Source: CAD feature listing. Evaluate the final solid. Frame: model axes, mm. Face numbers are marked on the shaded views. A direction names the side the tool comes from. Give positions to 0.01 mm unless a question says otherwise; leave off trailing zeros. Write item = value, one per line.
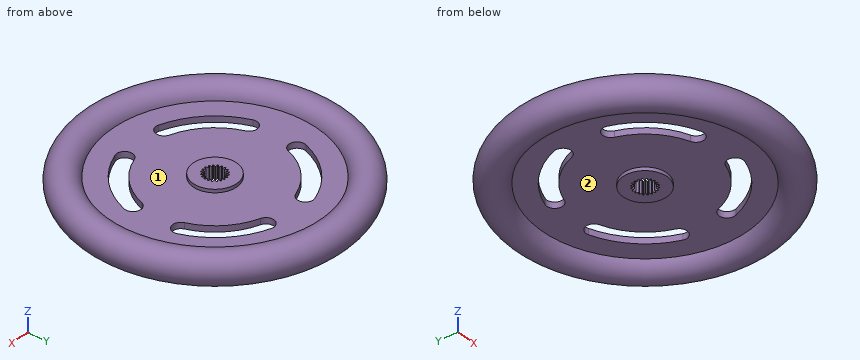
from build123d import *

# Parameters (mm, degrees)
SKETCH2_R                = 3.81
BOSS_EXTRUDE1_DEPTH      = 1.585
BOSS_EXTRUDE1_DEPTH_BACK = 1.585
SKETCH4_R                = 5.485
BOSS_EXTRUDE2_DEPTH      = 0.75
BOSS_EXTRUDE2_DEPTH_BACK = 0.75
SKETCH5_R                = 26.708345462
SKETCH5_R_2              = 4.443835797


with BuildPart() as part:
    # Sweep1: sweep along a path in Sketch1
    with BuildLine(Plane.XY) as sweep1_path:
        CenterArc((0, 0), 29.5275, 0, 360)
    # Sketch2 → Sweep1 (sweep)
    with BuildSketch(Plane(origin=(0, 0, 0), x_dir=(1, 0, 0), z_dir=(0, 1, 0))):
        with Locations((-29.5275, 0)):
            Circle(SKETCH2_R)
    sweep(path=sweep1_path.line)


with BuildPart() as body_2:
    # Sketch4 → Boss-Extrude1 (new, two sides: drawn at the far end of the back side and taken through both)
    with BuildSketch(Plane.XY.offset(-BOSS_EXTRUDE1_DEPTH_BACK)):
        with Locations((9.906, -10.287)):
            Circle(SKETCH4_R)
        with BuildLine():
            Line((9.502446481, -7.47395), (9.906, -8.063711559))
            Line((9.906, -8.063711559), (10.196958476, -7.460084913))
            ThreePointArc((10.196958476, -7.460084913), (10.294450159, -7.471824656), (10.391478053, -7.486925571))
            Line((10.391478053, -7.486925571), (10.593033912, -8.172527041))
            Line((10.593033912, -8.172527041), (11.056282758, -7.688355099))
            ThreePointArc((11.056282758, -7.688355099), (11.145375078, -7.729646845), (11.232987649, -7.773991937))
            Line((11.232987649, -7.773991937), (11.212816157, -8.488321868))
            Line((11.212816157, -8.488321868), (11.803009349, -8.170998754))
            ThreePointArc((11.803009349, -8.170998754), (11.87498133, -8.237800579), (11.944602449, -8.307049041))
            Line((11.944602449, -8.307049041), (11.704678132, -8.980183843))
            Line((11.704678132, -8.980183843), (12.364043448, -8.860771354))
            ThreePointArc((12.364043448, -8.860771354), (12.41184997, -8.94654423), (12.456664638, -9.03391754))
            Line((12.456664638, -9.03391754), (12.020472959, -9.599966088))
            Line((12.020472959, -9.599966088), (12.684467128, -9.690153151))
            ThreePointArc((12.684467128, -9.690153151), (12.703428556, -9.786501031), (12.71905, -9.883446481))
            Line((12.71905, -9.883446481), (12.129288441, -10.287))
            Line((12.129288441, -10.287), (12.732915087, -10.577958476))
            ThreePointArc((12.732915087, -10.577958476), (12.721175344, -10.675450159), (12.706074429, -10.772478053))
            Line((12.706074429, -10.772478053), (12.020472959, -10.974033912))
            Line((12.020472959, -10.974033912), (12.504644901, -11.437282758))
            ThreePointArc((12.504644901, -11.437282758), (12.463353155, -11.526375078), (12.419008063, -11.613987649))
            Line((12.419008063, -11.613987649), (11.704678132, -11.593816157))
            Line((11.704678132, -11.593816157), (12.022001246, -12.184009349))
            ThreePointArc((12.022001246, -12.184009349), (11.955199421, -12.25598133), (11.885950959, -12.325602449))
            Line((11.885950959, -12.325602449), (11.212816157, -12.085678132))
            Line((11.212816157, -12.085678132), (11.332228646, -12.745043448))
            ThreePointArc((11.332228646, -12.745043448), (11.24645577, -12.79284997), (11.15908246, -12.837664638))
            Line((11.15908246, -12.837664638), (10.593033912, -12.401472959))
            Line((10.593033912, -12.401472959), (10.502846849, -13.065467128))
            ThreePointArc((10.502846849, -13.065467128), (10.406498969, -13.084428556), (10.309553519, -13.10005))
            Line((10.309553519, -13.10005), (9.906, -12.510288441))
            Line((9.906, -12.510288441), (9.615041524, -13.113915087))
            ThreePointArc((9.615041524, -13.113915087), (9.517549841, -13.102175344), (9.420521947, -13.087074429))
            Line((9.420521947, -13.087074429), (9.218966088, -12.401472959))
            Line((9.218966088, -12.401472959), (8.755717242, -12.885644901))
            ThreePointArc((8.755717242, -12.885644901), (8.666624922, -12.844353155), (8.579012351, -12.800008063))
            Line((8.579012351, -12.800008063), (8.599183843, -12.085678132))
            Line((8.599183843, -12.085678132), (8.008990651, -12.403001246))
            ThreePointArc((8.008990651, -12.403001246), (7.93701867, -12.336199421), (7.867397551, -12.266950959))
            Line((7.867397551, -12.266950959), (8.107321868, -11.593816157))
            Line((8.107321868, -11.593816157), (7.447956552, -11.713228646))
            ThreePointArc((7.447956552, -11.713228646), (7.40015003, -11.62745577), (7.355335362, -11.54008246))
            Line((7.355335362, -11.54008246), (7.791527041, -10.974033912))
            Line((7.791527041, -10.974033912), (7.127532872, -10.883846849))
            ThreePointArc((7.127532872, -10.883846849), (7.108571444, -10.787498969), (7.09295, -10.690553519))
            Line((7.09295, -10.690553519), (7.682711559, -10.287))
            Line((7.682711559, -10.287), (7.079084913, -9.996041524))
            ThreePointArc((7.079084913, -9.996041524), (7.090824656, -9.898549841), (7.105925571, -9.801521947))
            Line((7.105925571, -9.801521947), (7.791527041, -9.599966088))
            Line((7.791527041, -9.599966088), (7.307355099, -9.136717242))
            ThreePointArc((7.307355099, -9.136717242), (7.348646845, -9.047624922), (7.392991937, -8.960012351))
            Line((7.392991937, -8.960012351), (8.107321868, -8.980183843))
            Line((8.107321868, -8.980183843), (7.789998754, -8.389990651))
            ThreePointArc((7.789998754, -8.389990651), (7.856800579, -8.31801867), (7.926049041, -8.248397551))
            Line((7.926049041, -8.248397551), (8.599183843, -8.488321868))
            Line((8.599183843, -8.488321868), (8.479771354, -7.828956552))
            ThreePointArc((8.479771354, -7.828956552), (8.56554423, -7.78115003), (8.65291754, -7.736335362))
            Line((8.65291754, -7.736335362), (9.218966088, -8.172527041))
            Line((9.218966088, -8.172527041), (9.309153151, -7.508532872))
            ThreePointArc((9.309153151, -7.508532872), (9.405501031, -7.489571444), (9.502446481, -7.47395))
        make_face(mode=Mode.SUBTRACT)
    extrude(amount=BOSS_EXTRUDE1_DEPTH + BOSS_EXTRUDE1_DEPTH_BACK)


with BuildPart() as body_3:
    # Sketch5 → Boss-Extrude2 (new, two sides: drawn at the far end of the back side and taken through both)
    with BuildSketch(Plane.XY.offset(-BOSS_EXTRUDE2_DEPTH_BACK)):
        Circle(SKETCH5_R)
        Circle(SKETCH5_R_2, mode=Mode.SUBTRACT)
        with BuildLine():
            ThreePointArc((19.605748825, 6.641704905), (14.637240707, 14.637240707), (6.641704905, 19.605748825))
            ThreePointArc((6.641704905, 19.605748825), (4.105741619, 18.353195349), (5.358295095, 15.817232063))
            ThreePointArc((5.358295095, 15.817232063), (11.808813583, 11.808813583), (15.817232063, 5.358295095))
            ThreePointArc((15.817232063, 5.358295095), (18.353195349, 4.105741619), (19.605748825, 6.641704905))
        make_face(mode=Mode.SUBTRACT)
        with BuildLine():
            ThreePointArc((-6.641704905, 19.605748825), (-14.637240707, 14.637240707), (-19.605748825, 6.641704905))
            ThreePointArc((-19.605748825, 6.641704905), (-18.353195349, 4.105741619), (-15.817232063, 5.358295095))
            ThreePointArc((-15.817232063, 5.358295095), (-11.808813583, 11.808813583), (-5.358295095, 15.817232063))
            ThreePointArc((-5.358295095, 15.817232063), (-4.105741619, 18.353195349), (-6.641704905, 19.605748825))
        make_face(mode=Mode.SUBTRACT)
        with BuildLine():
            ThreePointArc((6.641704905, -19.605748825), (14.637240707, -14.637240707), (19.605748825, -6.641704905))
            ThreePointArc((19.605748825, -6.641704905), (18.353195349, -4.105741619), (15.817232063, -5.358295095))
            ThreePointArc((15.817232063, -5.358295095), (11.808813583, -11.808813583), (5.358295095, -15.817232063))
            ThreePointArc((5.358295095, -15.817232063), (4.105741619, -18.353195349), (6.641704905, -19.605748825))
        make_face(mode=Mode.SUBTRACT)
        with BuildLine():
            ThreePointArc((-19.605748825, -6.641704905), (-14.637240707, -14.637240707), (-6.641704905, -19.605748825))
            ThreePointArc((-6.641704905, -19.605748825), (-4.105741619, -18.353195349), (-5.358295095, -15.817232063))
            ThreePointArc((-5.358295095, -15.817232063), (-11.808813583, -11.808813583), (-15.817232063, -5.358295095))
            ThreePointArc((-15.817232063, -5.358295095), (-18.353195349, -4.105741619), (-19.605748825, -6.641704905))
        make_face(mode=Mode.SUBTRACT)
    extrude(amount=BOSS_EXTRUDE2_DEPTH + BOSS_EXTRUDE2_DEPTH_BACK)


with BuildPart() as body_2_1:
    # Body-Move/Copy1: read off the stored shape, not the designer's step
    # Body-Move/Copy1: moved
    add(body_2.part.moved(Location((-9.906, 10.287, 0))))


with BuildPart() as body_3_1:
    add(body_3.part)

    # Combine3: union body 2, part
    add(body_2_1.part)
    add(part.part)


solid = body_3_1.part
1) Contact query for flat-ended pins moving along their axis: pin 1 (4 mm diameter, centred on x = 1.5, z = -0.5, fed in from -Y); pin 2 (12 mm diameter, centred on x = 1.5, y = 1, fed in from -Z) (3 decimals); pin 3 (10 mm diameter, centred on x = -22, y = 8, fed in from +Z). Output: stop coordinate, or through.
Computed:
pin_1 = -33.34
pin_2 = -1.585
pin_3 = 3.64
2) Access query for the marked faces 1 and 2. Directions: +Z, -Z, +X, -X, +Y, -Y. A direction counts if a zero-diameter tool reaches every point of the face in a straight line with its end or side. Return the directions, or none.
Computed:
face_1 = +Z
face_2 = -Z
3) Material intervals for L1, parallel to X at y = -12.5, z = 0.5; L2, parallel to Y at x = -5.5, z = 0; L3, parallel to Z at x = -0.5, y = -22.5, sorted ascending.
Computed:
L1 = -30.87 to -16.5, -11.07 to 11.07, 16.5 to 30.87
L2 = -32.88 to -19.65, -15.77 to 15.77, 19.65 to 32.88
L3 = -0.75 to 0.75
4) Cut plane A-A (x = 11). State how many separate pieces and enclosed holes the cut face has, then the cut area to 3 significant figures.
Computed:
separate_pieces = 3
enclosed_holes = 0
area = 153 mm²
